```python
from build123d import *

# Parameters (mm, degrees)
EXTRUDE1_DEPTH                        = 44.45
CHAMFER1_SIZE                         = 2.54
CHAMFER2_SIZE                         = 2.54
F_13_16_0_8125_DIAMETER_HOLE1_D       = 20.6375
F_13_16_0_8125_DIAMETER_HOLE1_DEPTH   = 63.754
F_1_2_20_TAPPED_HOLE1_D               = 11.50874
F_1_2_20_TAPPED_HOLE1_DEPTH           = 82.55
F_1_2_20_TAPPED_HOLE1_TIP             = 3.322287069
F_60_0_04_DIAMETER_HOLE1_REACH        = 46.45
F_60_0_04_DIAMETER_HOLE1_BORE_R       = 0.508
F_1_4_20_TAPPED_HOLE1_D               = 5.1054
F_1_4_0_25_DIAMETER_HOLE2_D           = 6.36778
F_1_4_0_25_DIAMETER_HOLE2_DEPTH       = 12.7
F_1_4_0_25_DIAMETER_HOLE2_CSINK_D     = 9.652
F_1_4_0_25_DIAMETER_HOLE2_CSINK_ANGLE = 90
F_1_4_0_25_DIAMETER_HOLE2_TIP         = 1.913074116
EXTRUDE4_DEPTH                        = 12.7
CHAMFER3_SIZE                         = 1.524
EXTRUDE5_DEPTH                        = 33.131


with BuildPart() as part:
    # Sketch1 → Extrude1 (new body)
    with BuildSketch(Plane.XY):
        Polygon((-63.5, 19.16234013), (-25.4, 19.16234013), (-25.4, 190.23134013), (0, 190.23134013), (0, -12.96865987), (-63.5, -12.96865987), align=None)
    extrude1 = extrude(amount=EXTRUDE1_DEPTH)

    # Mirror2: Extrude1 across plane
    add(extrude1.mirror(Plane(origin=(0, -12.96865987, 44.45), x_dir=(0, 0, 1), z_dir=(-1, 0, 0))))

    # Chamfer1
    chamfer1_edges = [part.edges().sort_by_distance(p)[0] for p in [
        (63.5, 19.16234013, 22.225),
        (25.4, 190.23134013, 22.225),
    ]]
    chamfer(chamfer1_edges, length=CHAMFER1_SIZE)

    # Chamfer2
    chamfer2_edges = [part.edges().sort_by_distance(p)[0] for p in [
        (-63.5, 19.16234013, 22.225),
        (-25.4, 190.23134013, 22.225),
    ]]
    chamfer(chamfer2_edges, length=CHAMFER2_SIZE)

    # 13/16 (0.8125) Diameter Hole1
    with Locations(Plane(origin=(0, 190.23134013, 24.511), x_dir=(0, 0, 1), z_dir=(0, 1, 0))):
        with Locations((0, 0)):
            Hole(F_13_16_0_8125_DIAMETER_HOLE1_D / 2, depth=F_13_16_0_8125_DIAMETER_HOLE1_DEPTH)

    # 1/2-20 Tapped Hole1
    with Locations(Plane(origin=(0, 126.47734013, 24.511), x_dir=(0, 0, 1), z_dir=(0, 1, 0))):
        with Locations((0, 0)):
            Hole(F_1_2_20_TAPPED_HOLE1_D / 2, depth=F_1_2_20_TAPPED_HOLE1_DEPTH)
            with Locations((0, 0, -(F_1_2_20_TAPPED_HOLE1_DEPTH + F_1_2_20_TAPPED_HOLE1_TIP / 2))):  # 120° drill point
                Cone(0, F_1_2_20_TAPPED_HOLE1_D / 2, F_1_2_20_TAPPED_HOLE1_TIP, mode=Mode.SUBTRACT)

    # #60 (0.04) Diameter Hole1 bore → #60 (0.04) Diameter Hole1 (cut, up to next)
    with BuildSketch(Plane.XY.offset(44.45), mode=Mode.PRIVATE) as f_60_0_04_diameter_hole1_sk1:
        with Locations((0, 129.27134013)):
            Circle(F_60_0_04_DIAMETER_HOLE1_BORE_R)
    f_60_0_04_diameter_hole1_tool1 = extrude(f_60_0_04_diameter_hole1_sk1.sketch, amount=-F_60_0_04_DIAMETER_HOLE1_REACH, mode=Mode.PRIVATE) & part.part
    add(f_60_0_04_diameter_hole1_tool1.solids().sort_by_distance((0, 129.27134, 44.45))[0], mode=Mode.SUBTRACT)

    # 1/4-20 Tapped Hole1 (through all)
    with Locations(Plane(origin=(0, 0, 0), x_dir=(-1, 0, 0), z_dir=(0, 0, -1))):
        with Locations((-25.4, 3.09684013), (25.4, 3.09684013)):
            Hole(F_1_4_20_TAPPED_HOLE1_D / 2)

    # 1/4 (0.25) Diameter Hole2
    with Locations(Plane(origin=(0, 0, 0), x_dir=(-1, 0, 0), z_dir=(0, 0, -1))):
        with Locations((-9.525, 3.09684013)):
            CounterSinkHole(F_1_4_0_25_DIAMETER_HOLE2_D / 2, F_1_4_0_25_DIAMETER_HOLE2_CSINK_D / 2, depth=F_1_4_0_25_DIAMETER_HOLE2_DEPTH, counter_sink_angle=F_1_4_0_25_DIAMETER_HOLE2_CSINK_ANGLE)
            with Locations((0, 0, -(F_1_4_0_25_DIAMETER_HOLE2_DEPTH + F_1_4_0_25_DIAMETER_HOLE2_TIP / 2))):  # 118° drill point
                Cone(0, F_1_4_0_25_DIAMETER_HOLE2_D / 2, F_1_4_0_25_DIAMETER_HOLE2_TIP, mode=Mode.SUBTRACT)

    # Sketch23 → Extrude4 (cut)
    with BuildSketch(Plane(origin=(0, 0, 0), x_dir=(-1, 0, 0), z_dir=(0, 0, -1))):
        with BuildLine():
            Line((6.35, 6.28073013), (12.7, 6.28073013))
            ThreePointArc((12.7, 6.28073013), (15.88389, 3.09684013), (12.7, -0.08704987))
            Line((12.7, -0.08704987), (6.35, -0.08704987))
            ThreePointArc((6.35, -0.08704987), (3.16611, 3.09684013), (6.35, 6.28073013))
        make_face()
    extrude(amount=-EXTRUDE4_DEPTH, mode=Mode.SUBTRACT)

    # Chamfer3
    chamfer3_edges = [part.edges().sort_by_distance(p)[0] for p in [
        (-3.16611, 3.09684013, 0),
        (-9.525, -0.08704987, 0),
        (-15.88389, 3.09684013, 0),
        (-9.525, 6.28073013, 0),
    ]]
    chamfer(chamfer3_edges, length=CHAMFER3_SIZE)

    # Sketch24 → Extrude5 (cut, through all)
    with BuildSketch(Plane(origin=(0, 19.16234013, 0), x_dir=(1, 0, 0), z_dir=(0, 1, 0))):
        with BuildLine():
            Line((45.183374064, -15.7226), (50.009374064, -15.7226))
            ThreePointArc((50.009374064, -15.7226), (57.146774064, -22.86), (50.009374064, -29.9974))
            Line((50.009374064, -29.9974), (45.183374064, -29.9974))
            ThreePointArc((45.183374064, -29.9974), (38.045974064, -22.86), (45.183374064, -15.7226))
        make_face()
        with BuildLine():
            Line((-38.255625936, -29.9974), (-63.655625936, -29.9974))
            ThreePointArc((-63.655625936, -29.9974), (-70.793025936, -22.86), (-63.655625936, -15.7226))
            Line((-63.655625936, -15.7226), (-38.255625936, -15.7226))
            ThreePointArc((-38.255625936, -15.7226), (-31.118225936, -22.86), (-38.255625936, -29.9974))
        make_face()
    extrude(amount=-EXTRUDE5_DEPTH, mode=Mode.SUBTRACT)


solid = part.part
```
Part model, mm, in its own coordinate system. A direction names the side the tool comes from. Round coordinates to 2 decimals unless told otherwise and drop trailing zeros. Write each loop counter-clockwise with the first axis right and the second up, starting at its lowest first coordinate (ties: lowest second). Pieces come first, ordered by that corner, then holes.
Item 1: Which spindle directions (+Z, -Z, +X, -X, +Y, -Y) get a long thin tool onto all of the face, cutting with end or side? Do faces 4 (the cylindrical face through (57.145, 3.322, 22.703)), 5 (the flat face through (-9, 6.281, 7)), 6 (the flat face through (0, 190.231, 12)), 7 (the flat face through (39, 19.162, 17)), 8 (the flat face through (-25.4, 102, 22)). Say none if no direction does.
Results:
face 4: +Y, -Y
face 5: -Z
face 6: +Z, -Z, +X, -X, +Y
face 7: +Z, -Z, +X, +Y
face 8: +Z, -Z, -X, +Y
Item 2: Two-plate mould, pull along X, no slides. Class faces 1 (the flat face through (-63.5, 2, 8)), 2 (the flat face through (-10, 3, 12.7)), 3 (the flat face through (-51, 3, 29.997)): +X half, -X half, draft (parallel to the pull), parting line (faces both ways), or undercut.
Results:
face 1: -X half
face 2: undercut
face 3: draft
Item 3: Cut at C-C, the plane z = 21. Count the separate pieces of the cut face and the enclosed holes in it, plus the area to 3 significant figures.
Results:
separate pieces: 2
enclosed holes: 2
area: 9,090 mm2
Item 4: Probe L1, parallel to Y at x = 0, z = 38; L2, parallel to Z at x = 0, y = 92.5; L3, parallel to X at y = 139, z = 24.5. List the from-to ranges inside material, lowest first.
Results:
L1: y = -12.97 to 128.76, 129.78 to 190.23
L2: z = 0 to 18.76, 30.27 to 44.45
L3: x = -25.4 to -10.32, 10.32 to 25.4
Item 5: Cut at B-B, the plane z = 5. Give the cut face in (x, y) (3 decimals).
Results:
outline: (-63.5, -12.969) - (63.5, -12.969) - (63.5, 16.622) - (60.96, 19.162) - (25.4, 19.162) - (25.4, 187.691) - (22.86, 190.231) - (-22.86, 190.231) - (-25.4, 187.691) - (-25.4, 19.162) - (-60.96, 19.162) - (-63.5, 16.622) - close; hole circle Ø5.105 at (-25.4, 3.097); hole (-12.7, -0.087) - (-6.35, -0.087) arc R3.184 ccw to (-6.35, 6.281) - (-12.7, 6.281) arc R3.184 ccw to start; hole circle Ø6.368 at (9.525, 3.097); hole circle Ø5.105 at (25.4, 3.097)
Item 6: Drop flat-ended pins along their axis: pin 1 Ø8 at (y, z) = (122.5, 13) entering from +X; pin 2 Ø10 at (y, z) = (122.5, 13.5) entering from -X; pin 3 Ø3 at (x, y) = (-9, 4) entering from -Z. Give the stop position or say it passes through.
Results:
pin 1: stops at x = 25.4
pin 2: stops at x = -25.4
pin 3: stops at z = 12.7
Item 7: Cut at A-A, the plane y = 49.5. Give the cut face in (x, z).
Results:
outline: (-25.4, 0) - (25.4, 0) - (25.4, 44.45) - (-25.4, 44.45) - close; hole circle Ø11.51 at (0, 24.51)
Item 8: Cut at D-D, the plane y = 148. Give the cut face in (x, z).
Results:
outline: (-25.4, 0) - (25.4, 0) - (25.4, 44.45) - (-25.4, 44.45) - close; hole circle Ø20.64 at (0, 24.51)
